Check sheet for the modelled part. Datum: model origin and axes. Units: mm. A direction names the side the tool comes from. Round coordinates to 2 decimals unless told otherwise and drop trailing zeros. Write each loop counter-clockwise with the first axis right and the second up, starting at its lowest first coordinate (ties: lowest second). Pieces come first, ordered by that corner, then holes.
Item 1: Go/stop test with flat-tipped pins: pin 1 Ø3 at (x, y) = (2, -77) entering from -Z (3 decimals); pin 2 Ø2 at (y, z) = (24.5, 1.5) entering from +X; pin 3 Ø6.5 at (x, z) = (-4.5, 9.5) entering from +Y (3 decimals). Record where each tip stops, or that it passes through.
Item 2: Material ranges on line 1 (X direction, y = -21, z = 8.75); line 2 (Y direction, x = -33, z = 8.25) (3 decimals); line 3 (Z direction, x = 2.5, y = 7), recorded low to high.
Item 3: Cross-section at A-A on x = -5.5. Count the separate pieces of the cut face and the enclosed holes in it, plus the area to 3 significant figures.
Item 4: Cross-section at B-B on y = 3.5. Enter the section's corners in (x, z) (1 decimal).
Item 5: Release check for a two-part mould opening along Y. For faces 1 (the flat face through (38.1, 1, 9)), 2 (the flat face through (32, 82.55, 8)), 3 (the flat face through (-42, 7, 15.875)), 4 (the flat face through (45, 20, 7.938)) record: +Y half, -Y half, draft (parallel to the pull), parting line (faces both ways), or undercut.
Item 6: Cross-section at C-C on z = 4.5. Enter the section's corners in (x, y) (3 decimals).
Item 7: Tool access check on faces 5 (the flat face through (9.525, -78, 5)), 6 (the flat face through (-1, -82.55, 10)), 7 (the flat face through (0, -78, 9.525)), 8 (the flat face through (25, 73.025, 9)), 9 (the flat face through (-12.7, 78, 8)). Record the directions out of +Z, -Z, +X, -X, +Y, -Y that give a thin tool (end or side, any length) a straight path to the whole face; none if there is none.
from build123d import *

# Parameters (mm, degrees)
F0_W      = 12.7
F0_H      = 9.525
F0_W_2    = 76.2
F0_H_2    = 146.05
F1_DEPTH  = 15.875
F2_DEPTH  = 2.54
F3_W      = 19.05
F3_H      = 9.525
F4_DEPTH  = 9.525
F5_W      = 41.275
F5_H      = 7.9375
F6_DEPTH  = 12.7
F7_W      = 20.32
F7_H      = 27.94
F8_DEPTH  = 25.4
F9_W      = 25.4
F9_H      = 15.875
F10_DEPTH = 12.7


with BuildPart() as f1:
    # F0 (on Top) → F1 (new body)
    with BuildSketch(Plane.XY):
        with Locations((44.45, 77.7875)):
            Rectangle(F0_W, F0_H)
        with Locations((-44.45, 77.7875)):
            Rectangle(F0_W, F0_H)
        with Locations((44.45, -77.7875)):
            Rectangle(F0_W, F0_H)
        with Locations((0, -77.7875)):
            Rectangle(F0_W_2, F0_H)
        with Locations((44.45, 0)):
            Rectangle(F0_W, F0_H_2)
        with Locations((-44.45, -77.7875)):
            Rectangle(F0_W, F0_H)
        with Locations((-44.45, 0)):
            Rectangle(F0_W, F0_H_2)
        with Locations((0, 77.7875)):
            Rectangle(F0_W_2, F0_H)
    extrude(amount=F1_DEPTH)

    # F0 (on Top) → F2 (join)
    with BuildSketch(Plane.XY):
        Rectangle(F0_W_2, F0_H_2)
    extrude(amount=F2_DEPTH)

    # F3 (on face) → F4 (cut)
    with BuildSketch(Plane.XZ.offset(82.55)):
        with Locations((0, 4.7625)):
            Rectangle(F3_W, F3_H)
    extrude(amount=-F4_DEPTH, mode=Mode.SUBTRACT)

    # F5 (on face) → F6 (cut)
    with BuildSketch(Plane.YZ.offset(50.8)):
        with Locations((20.6375, 3.96875)):
            Rectangle(F5_W, F5_H)
    extrude(amount=-F6_DEPTH, mode=Mode.SUBTRACT)

    # F7 (on face) → F8 (cut)
    with BuildSketch(Plane(origin=(0, 0, 0), x_dir=(1, 0, 0), z_dir=(0, 0, -1))):
        with Locations((0, -47.9425)):
            Rectangle(F7_W, F7_H)
    extrude(amount=-F8_DEPTH, mode=Mode.SUBTRACT)

    # F9 (on face) → F10 (cut)
    with BuildSketch(Plane(origin=(0, 82.55, 0), x_dir=(-1, 0, 0), z_dir=(0, 1, 0))):
        with Locations((0, 7.9375)):
            Rectangle(F9_W, F9_H)
    extrude(amount=-F10_DEPTH, mode=Mode.SUBTRACT)


solid = f1.part
Response values:
1. pin 1: stops at z = 9.525
1. pin 2: stops at x = 38.1
1. pin 3: stops at y = -73.025
2. line 1: x = -50.8 to -38.1, 38.1 to 50.8
2. line 2: y = -82.55 to -73.025, 73.025 to 82.55
2. line 3: z = 0 to 2.54
3. separate pieces: 3
3. enclosed holes: 0
3. area: 352 mm2
4. outline: (-50.8, 0) - (38.1, 0) - (38.1, 2.5) - (-38.1, 2.5) - (-38.1, 15.9) - (-50.8, 15.9) - close; (38.1, 7.9) - (50.8, 7.9) - (50.8, 15.9) - (38.1, 15.9) - close
5. face 1: undercut
5. face 2: +Y half
5. face 3: draft
5. face 4: undercut
6. outline: (-50.8, -82.55) - (-9.525, -82.55) - (-9.525, -73.025) - (-38.1, -73.025) - (-38.1, 73.025) - (-12.7, 73.025) - (-12.7, 82.55) - (-50.8, 82.55) - close; (9.525, -82.55) - (50.8, -82.55) - (50.8, 0) - (38.1, 0) - (38.1, -73.025) - (9.525, -73.025) - close; (12.7, 73.025) - (38.1, 73.025) - (38.1, 41.275) - (50.8, 41.275) - (50.8, 82.55) - (12.7, 82.55) - close
7. face 5: -Z, -Y
7. face 6: +Z, -Z, +X, -X, -Y
7. face 7: -Z, +Y, -Y
7. face 8: +Z
7. face 9: +Z, -Z, +Y
